```python
from build123d import *

# Parameters (mm, degrees)
SKETCH2_R           = 1.7
BOSS_EXTRUDE1_DEPTH = 10
BOSS_EXTRUDE2_DEPTH = 10
SKETCH3_R           = 1.7
CUT_EXTRUDE1_DEPTH  = 72.091490349


with BuildPart() as part:
    # Sketch2 → Boss-Extrude1 (new body)
    with BuildSketch(Plane(origin=(0, 0, 0), x_dir=(1, 0, 0), z_dir=(0, 1, 0))):
        with BuildLine():
            ThreePointArc((60, -5), (65, 0), (60, 5))
            Line((60, 5), (21.937410968, 5))
            ThreePointArc((21.937410968, 5), (20.937955519, 8.237233678), (19.463757806, 11.287698262))
            ThreePointArc((19.463757806, 11.287698262), (21.232218388, 13.021454794), (22.284297787, 15.263439066))
            Line((22.284297787, 15.263439066), (21.402619909, 16.476964558))
            ThreePointArc((21.402619909, 16.476964558), (18.945255744, 16.16918883), (16.749870923, 15.023043103))
            ThreePointArc((16.749870923, 15.023043103), (15.909902577, 15.909902577), (15.023043103, 16.749870923))
            ThreePointArc((15.023043103, 16.749870923), (16.16918883, 18.945255744), (16.476964558, 21.402619909))
            Line((16.476964558, 21.402619909), (15.263439066, 22.284297787))
            ThreePointArc((15.263439066, 22.284297787), (13.021454794, 21.232218388), (11.287698262, 19.463757806))
            ThreePointArc((11.287698262, 19.463757806), (10.214786244, 20.047646794), (9.111768269, 20.572449514))
            ThreePointArc((9.111768269, 20.572449514), (9.523406413, 23.014563062), (9.056751235, 25.446763194))
            Line((9.056751235, 25.446763194), (7.630166461, 25.910288686))
            ThreePointArc((7.630166461, 25.910288686), (5.823023123, 24.216890476), (4.72060705, 21.999224284))
            ThreePointArc((4.72060705, 21.999224284), (3.519775463, 22.222987663), (2.308570071, 22.381253411))
            ThreePointArc((2.308570071, 22.381253411), (1.945406622, 24.831044595), (0.75, 27))
            Line((0.75, 27), (-0.75, 27))
            ThreePointArc((-0.75, 27), (-1.945406622, 24.831044595), (-2.308570071, 22.381253411))
            ThreePointArc((-2.308570071, 22.381253411), (-3.519775463, 22.222987663), (-4.72060705, 21.999224284))
            ThreePointArc((-4.72060705, 21.999224284), (-5.823023123, 24.216890476), (-7.630166461, 25.910288686))
            Line((-7.630166461, 25.910288686), (-9.056751235, 25.446763194))
            ThreePointArc((-9.056751235, 25.446763194), (-9.523406413, 23.014563062), (-9.111768269, 20.572449514))
            ThreePointArc((-9.111768269, 20.572449514), (-10.214786244, 20.047646794), (-11.287698262, 19.463757806))
            ThreePointArc((-11.287698262, 19.463757806), (-13.021454794, 21.232218388), (-15.263439066, 22.284297787))
            Line((-15.263439066, 22.284297787), (-16.476964558, 21.402619909))
            ThreePointArc((-16.476964558, 21.402619909), (-16.16918883, 18.945255744), (-15.023043103, 16.749870923))
            ThreePointArc((-15.023043103, 16.749870923), (-15.909902577, 15.909902577), (-16.749870923, 15.023043103))
            ThreePointArc((-16.749870923, 15.023043103), (-18.945255744, 16.16918883), (-21.402619909, 16.476964558))
            Line((-21.402619909, 16.476964558), (-22.284297787, 15.263439066))
            ThreePointArc((-22.284297787, 15.263439066), (-21.232218388, 13.021454794), (-19.463757806, 11.287698262))
            ThreePointArc((-19.463757806, 11.287698262), (-20.047646794, 10.214786244), (-20.572449514, 9.111768269))
            ThreePointArc((-20.572449514, 9.111768269), (-23.014563062, 9.523406413), (-25.446763194, 9.056751235))
            Line((-25.446763194, 9.056751235), (-25.910288686, 7.630166461))
            ThreePointArc((-25.910288686, 7.630166461), (-24.216890476, 5.823023123), (-21.999224284, 4.72060705))
            ThreePointArc((-21.999224284, 4.72060705), (-22.222987663, 3.519775463), (-22.381253411, 2.308570071))
            ThreePointArc((-22.381253411, 2.308570071), (-24.831044595, 1.945406622), (-27, 0.75))
            Line((-27, 0.75), (-27, -0.75))
            ThreePointArc((-27, -0.75), (-24.831044595, -1.945406622), (-22.381253411, -2.308570071))
            ThreePointArc((-22.381253411, -2.308570071), (-22.222987663, -3.519775463), (-21.999224284, -4.72060705))
            ThreePointArc((-21.999224284, -4.72060705), (-24.216890476, -5.823023123), (-25.910288686, -7.630166461))
            Line((-25.910288686, -7.630166461), (-25.446763194, -9.056751235))
            ThreePointArc((-25.446763194, -9.056751235), (-23.014563062, -9.523406413), (-20.572449514, -9.111768269))
            ThreePointArc((-20.572449514, -9.111768269), (-20.047646794, -10.214786244), (-19.463757806, -11.287698262))
            ThreePointArc((-19.463757806, -11.287698262), (-21.232218388, -13.021454794), (-22.284297787, -15.263439066))
            Line((-22.284297787, -15.263439066), (-21.402619909, -16.476964558))
            ThreePointArc((-21.402619909, -16.476964558), (-18.945255744, -16.16918883), (-16.749870923, -15.023043103))
            ThreePointArc((-16.749870923, -15.023043103), (-15.909902577, -15.909902577), (-15.023043103, -16.749870923))
            ThreePointArc((-15.023043103, -16.749870923), (-16.16918883, -18.945255744), (-16.476964558, -21.402619909))
            Line((-16.476964558, -21.402619909), (-15.263439066, -22.284297787))
            ThreePointArc((-15.263439066, -22.284297787), (-13.021454794, -21.232218388), (-11.287698262, -19.463757806))
            ThreePointArc((-11.287698262, -19.463757806), (9.111768269, -20.572449514), (21.999224284, -4.72060705))
            ThreePointArc((21.999224284, -4.72060705), (22.395016771, -4.848633199), (22.782483518, -5))
            Line((22.782483518, -5), (60, -5))
        make_face()
        with BuildLine():
            ThreePointArc((22.381253411, 2.308570071), (24.831044595, 1.945406622), (27, 0.75))
            Line((27, 0.75), (27, -0.75))
            ThreePointArc((27, -0.75), (24.831044595, -1.945406622), (22.381253411, -2.308570071))
            ThreePointArc((22.381253411, -2.308570071), (22.5, 0), (22.381253411, 2.308570071))
        make_face(mode=Mode.SUBTRACT)
        with Locations(Location((60, 0, 0), (0, 0, 270))):
            Circle(SKETCH2_R, mode=Mode.SUBTRACT)
    extrude(amount=BOSS_EXTRUDE1_DEPTH)

    # Sketch2<7> → Boss-Extrude2 (add)
    with BuildSketch(Plane(origin=(0, 0, 0), x_dir=(1, 0, 0), z_dir=(0, 1, 0))):
        with BuildLine():
            Line((21.937410968, -5), (22.782483518, -5))
            ThreePointArc((22.782483518, -5), (22.395016771, -4.848633199), (21.999224284, -4.72060705))
            ThreePointArc((21.999224284, -4.72060705), (21.968761786, -4.860401792), (21.937410968, -5))
        make_face()
        with BuildLine():
            ThreePointArc((27, 0.75), (24.831044595, 1.945406622), (22.381253411, 2.308570071))
            ThreePointArc((22.381253411, 2.308570071), (22.5, 0), (22.381253411, -2.308570071))
            ThreePointArc((22.381253411, -2.308570071), (24.831044595, -1.945406622), (27, -0.75))
            Line((27, -0.75), (27, 0.75))
        make_face()
    extrude(amount=BOSS_EXTRUDE2_DEPTH)

    # Sketch3 → Cut-Extrude1 (cut, through all)
    with BuildSketch(Plane(origin=(0, 10, 0), x_dir=(1, 0, 0), z_dir=(0, 1, 0))):
        with Locations(Location((0, 0, 0), (0, 0, 270))):
            Circle(SKETCH3_R)
    extrude(amount=-CUT_EXTRUDE1_DEPTH, mode=Mode.SUBTRACT)


solid = part.part
```
The listing builds one solid part. Answer for the finished solid, in the listing's coordinates (mm). A direction names the side the tool comes from. Coordinates: 2 decimals unless noted, no trailing zeros. Loops run counter-clockwise (first coordinate to the right, second up) from the corner with the lowest first, then second, coordinate; pieces in that order, holes last. Notation, with made-up numbers: (12, 83.5) -> (46, 83.5) arc R11 cw to (46, 90.5) -> close; hole circle Ø4 at (-13.75, 74). An arc over 180 degrees is marked (long way). Use one line per item in the form item = value. Start each with the question number.
Item 1: The mould has two halves that part along Z. Classify faces 6 (the face through (-3.503, 4.93, -22.226)), 7 (the face through (-21.25, 4.93, -13.05)), 8 (the face through (20.955, 4.93, -8.193)), 9 (the face through (8.71, 4.93, 20.746)): released by +Z, released by -Z, zero draft, split by the parting line, or undercut.
Item 2: The part is cut by section B-B on y = 1.5. Count the separate pieces of the cut face and the enclosed holes in it, then the cut area to 3 significant figures.
Item 3: The part is cut by section A-A on x = 30. Determine the outline of the cut face in (y, z), then the cut area to 3 significant figures.
Item 4: A tool of negligible diameter and unlimited length cuts with its end or side. For faces 1 (the face through (13.05, 4.93, -21.25)), 2 (the face through (21.21, 4.93, -12.99)), 3 (the face through (41, 5, 5)), 4 (the face through (-22.226, 4.93, 3.503)), 5 (the face through (15.92, 4.93, -15.9)), from which of +Z, -Z, +X, -X, +Y, -Y can it reach the whole face along a straight path? Write none if from no direction.
Item 5: Consider L1, parallel to X at y = 7.5, z = 0; L2, parallel to Z at x = 35, y = 4.75; L3, parallel to X at y = 3.25, z = 1.5. Determine where each line is inside the solid, lowest interval first. Write a range as [from, to].
Item 6: Flat-ended cylindrical pins translate along their axes: pin 1 Ø4 at (x, y) = (14, 3.5) entering from -Z; pin 2 Ø6 at (x, y) = (32, 5.5) entering from +Z; pin 3 Ø3 at (x, y) = (36, 3.5) entering from -Z. Find the tip coordinate at first contact, or state that the pin passes through.
Item 7: The part is cut by section C-C on z = -6.5. Determine the outline of the cut face in (x, y), then the cut area to 3 significant figures.
Answer key:
q1.face_6 = released by -Z
q1.face_7 = undercut
q1.face_8 = undercut
q1.face_9 = released by +Z
q2.separate_pieces = 1
q2.enclosed_holes = 2
q2.area = 2,190 mm2
q3.outline = (0, -5) -> (10, -5) -> (10, 5) -> (0, 5) -> close
q3.area = 100 mm2
q4.face_1 = -Z, +Y, -Y
q4.face_2 = +X, +Y, -Y
q4.face_3 = +Z, +X, +Y, -Y
q4.face_4 = -X, +Y, -Y
q4.face_5 = +Y, -Y
q5.L1 = [-27, -1.7], [1.7, 58.3], [61.7, 65]
q5.L2 = [-5, 5]
q5.L3 = [-25.87, -0.8], [0.8, 59.2], [60.8, 64.77]
q6.pin_1 = -22.28
q6.pin_2 = 5
q6.pin_3 = -5
q7.outline = (-25, 0) -> (21.54, 0) -> (21.54, 10) -> (-25, 10) -> close
q7.area = 465 mm2
